Part model, mm, in its own coordinate system. A direction names the side the tool comes from. Round coordinates to 2 decimals unless told otherwise and drop trailing zeros. Loops run counter-clockwise (first coordinate to the right, second up) from the corner with the lowest first, then second, coordinate; pieces in that order, holes last. Notation, with made-up numbers: (27, 46.5) -> (86, 46.5) arc R15 ccw to (86, 50.5) -> close; hole circle Ø3 at (27, -25.5). An arc over 180 degrees is marked (long way). Use a Markdown table: item, result. Add a question column.
Item 1: Cut at D-D, the plane z = 0. State how many separate pieces and enclosed holes the cut face has, plus the area to 3 significant figures.
Item 2: Flat gauge pins, fed straight in: pin 1 (2 mm diameter, centred on x = 10.5, z = -0.5, fed in from +Y); pin 2 (8 mm diameter, centred on y = 8, z = 10.5, fed in from +X); pin 3 (2 mm diameter, centred on y = 11.5, z = 0.5, fed in from -X). Where does each tip first touch, or does it go through?
Item 3: Cut at B-B, the plane x = -10.25. List the corners of the cut face in (y, z), plus the area to 3 significant figures.
Item 4: Cut at C-C, the plane y = 23.5. List the corners of the cut face in (x, z), plus the area to 3 significant figures.
Item 5: Which spindle directions (+Z, -Z, +X, -X, +Y, -Y) get a long thin tool onto all of the face, cutting with end or side? Do faces 4 (the face through (-5, 2.2, 9)), 5 (the face through (-3.905, 10.507, 0.867)), 6 (the face through (0, 0, 0)), 7 (the face through (-7.5, 11, 0)), 8 (the face through (-4.28, 2, 9.91)). Say none if no direction does.
Item 6: Probe line 1 (X direction, y = 2.1, z = 0); line 2 (Z direction, x = 0, y = 2.15); line 3 (Y direction, x = 3.75, z = -1.25). List the from-to ranges inside material, lowest first. Write a range as [from, to].
Item 7: Cut at A-A, the plane y = 10.5. List the corners of the cut face in (x, z).
Item 8: Two-plate mould, pull along X, no slides. Class faces 1 (the face through (9.6, 1.8, 0)), 2 (the face through (-6.46, 2, 8.69)), 3 (the face through (10.75, 2, -0.02)): pulls with the +X half, pulls with the -X half, needs draft (parallel to the pull), parting line crosses it, or undercut.
```python
from build123d import *

# Parameters (mm, degrees)
SKETCH2_W           = 0.4
SKETCH2_H           = 2.8
BOSS_EXTRUDE1_DEPTH = 2.5
SKETCH3_R           = 0.5
BOSS_EXTRUDE2_DEPTH = 0.2
SKETCH4_R           = 3
BOSS_EXTRUDE4_DEPTH = 15
CUT_EXTRUDE1_DEPTH  = 12
CHAMFER1_SIZE       = 0.5


with BuildPart() as part:
    # Sketch1 → Revolve1 (revolve)
    with BuildSketch(Plane(origin=(0, 0, 0), x_dir=(0, 0, -1), z_dir=(1, 0, 0))):
        Polygon((0, 0), (8.5, 0), (8.5, 10), (4, 10), (4, 11), (3.5, 11), (3.5, 16), (0, 16), align=None)
    revolve(axis=Axis((0, 16, 0), (0, -1, 0)))

    # Sketch2 → Boss-Extrude1 (add)
    with BuildSketch(Plane(origin=(0, 10, 0), x_dir=(1, 0, 0), z_dir=(0, 1, 0))):
        with Locations((-7.3, 0)):
            Rectangle(SKETCH2_W, SKETCH2_H)
    extrude(amount=BOSS_EXTRUDE1_DEPTH)

    # Sketch3 → Boss-Extrude2 (add, symmetric)
    with BuildSketch(Plane(origin=(0, 2, 0), x_dir=(-1, 0, 0), z_dir=(0, -1, 0))):
        with BuildLine():
            Line((-1.25, -9.485281374), (-1.25, -12))
            ThreePointArc((-1.25, -12), (0, -13.25), (1.25, -12))
            Line((1.25, -12), (1.25, -9.485281374))
            Line((1.25, -9.485281374), (0.5, -9.485281374))
            Line((0.5, -9.485281374), (0.5, -8.485281374))
            ThreePointArc((0.5, -8.485281374), (0, -8.5), (-0.5, -8.485281374))
            Line((-0.5, -8.485281374), (-0.5, -9.485281374))
            Line((-0.5, -9.485281374), (-1.25, -9.485281374))
        make_face()
        with Locations((0, -12)):
            Circle(SKETCH3_R, mode=Mode.SUBTRACT)
        with BuildLine():
            Line((-5.825172442, -7.589494632), (-7.082531755, -9.767304845))
            ThreePointArc((-7.082531755, -9.767304845), (-6.625, -11.4748366), (-4.917468245, -11.017304845))
            Line((-4.917468245, -11.017304845), (-3.660108932, -8.839494632))
            Line((-3.660108932, -8.839494632), (-4.309627985, -8.464494632))
            Line((-4.309627985, -8.464494632), (-3.809627985, -7.598469228))
            ThreePointArc((-3.809627985, -7.598469228), (-4.25, -7.361215932), (-4.675653389, -7.098469228))
            Line((-4.675653389, -7.098469228), (-5.175653389, -7.964494632))
            Line((-5.175653389, -7.964494632), (-5.825172442, -7.589494632))
        make_face()
        with Locations((-6, -10.392304845)):
            Circle(SKETCH3_R, mode=Mode.SUBTRACT)
        with BuildLine():
            Line((5.175653389, -7.964494632), (4.675653389, -7.098469228))
            ThreePointArc((4.675653389, -7.098469228), (4.25, -7.361215932), (3.809627985, -7.598469228))
            Line((3.809627985, -7.598469228), (4.309627985, -8.464494632))
            Line((4.309627985, -8.464494632), (3.660108932, -8.839494632))
            Line((3.660108932, -8.839494632), (4.917468245, -11.017304845))
            ThreePointArc((4.917468245, -11.017304845), (6.625, -11.4748366), (7.082531755, -9.767304845))
            Line((7.082531755, -9.767304845), (5.825172442, -7.589494632))
            Line((5.825172442, -7.589494632), (5.175653389, -7.964494632))
        make_face()
        with Locations((6, -10.392304845)):
            Circle(SKETCH3_R, mode=Mode.SUBTRACT)
        with BuildLine():
            Line((9.383974596, 0.5), (8.485281374, 0.5))
            ThreePointArc((8.485281374, 0.5), (8.5, 0), (8.485281374, -0.5))
            Line((8.485281374, -0.5), (9.383974596, -0.5))
            ThreePointArc((9.383974596, -0.5), (11.25, 0), (9.383974596, 0.5))
        make_face()
        with Locations((10.25, 0)):
            Circle(SKETCH3_R, mode=Mode.SUBTRACT)
        with BuildLine():
            Line((-9.383974596, -0.5), (-8.485281374, -0.5))
            ThreePointArc((-8.485281374, -0.5), (-8.5, 0), (-8.485281374, 0.5))
            Line((-8.485281374, 0.5), (-9.383974596, 0.5))
            ThreePointArc((-9.383974596, 0.5), (-11.25, 0), (-9.383974596, -0.5))
        make_face()
        with Locations((-10.25, 0)):
            Circle(SKETCH3_R, mode=Mode.SUBTRACT)
    extrude(amount=BOSS_EXTRUDE2_DEPTH, both=True)

    # Sketch4 → Boss-Extrude4 (add)
    with BuildSketch(Plane(origin=(0, 16, 0), x_dir=(1, 0, 0), z_dir=(0, 1, 0))):
        Circle(SKETCH4_R)
    extrude(amount=BOSS_EXTRUDE4_DEPTH)

    # Sketch5 → Cut-Extrude1 (cut)
    with BuildSketch(Plane(origin=(0, 31, 0), x_dir=(1, 0, 0), z_dir=(0, 1, 0))):
        with BuildLine():
            Line((2.954423259, -0.520944533), (-1.02606043, 2.819077862))
            ThreePointArc((-1.02606043, 2.819077862), (1.928362829, 2.298133329), (2.954423259, -0.520944533))
        make_face()
    extrude(amount=-CUT_EXTRUDE1_DEPTH, mode=Mode.SUBTRACT)

    # Chamfer1
    chamfer1_edges = [part.edges().sort_by_distance(p)[0] for p in [
        (-1.928362829, 31, 2.298133329),
        (0.964181415, 31, -1.149066665),
    ]]
    chamfer(chamfer1_edges, length=CHAMFER1_SIZE)


solid = part.part
```
A:
| question | item | result |
|---|---|---|
| 1 | separate pieces | 3 |
| 1 | enclosed holes | 0 |
| 1 | area | 297 mm^2 |
| 2 | pin 1 | stops at y = 2.2 |
| 2 | pin 2 | stops at x = 5.48 |
| 2 | pin 3 | stops at x = -7.5 |
| 3 | outline | (1.8, -1) -> (2.2, -1) -> (2.2, -0.5) -> (1.8, -0.5) -> close; (1.8, 0.5) -> (2.2, 0.5) -> (2.2, 1) -> (1.8, 1) -> close |
| 3 | area | 0.400 mm^2 |
| 4 | outline | (-1.03, -2.82) -> (2.95, 0.52) arc R3 ccw (long way) to start |
| 4 | area | 22.7 mm^2 |
| 5 | face 4 | +Z, -X, +Y |
| 5 | face 5 | +Y |
| 5 | face 6 | +Z, -Z, +X, -X, -Y |
| 5 | face 7 | +Z, -Z, -X, +Y |
| 5 | face 8 | +Z, +Y, -Y |
| 6 | line 1 | x = [-11.25, -10.75], [-9.75, 9.75], [10.75, 11.25] |
| 6 | line 2 | z = [-8.5, 11.5], [12.5, 13.25] |
| 6 | line 3 | y = [0, 11] |
| 7 | outline | (-7.5, -1.4) -> (-7.1, -1.4) -> (-7.1, 1.4) -> (-7.5, 1.4) -> close; circle Ø8 at (0, 0) |
| 8 | face 1 | needs draft |
| 8 | face 2 | pulls with the -X half |
| 8 | face 3 | undercut |
